For this review, take the finished solid that the model builds, in its own axes (mm). A direction names the side the tool comes from. Give positions to 0.01 mm unless a question says otherwise; leave off trailing zeros. Order: outer loops, then holes, each group sorted by start corner. A loop starts at its lowest first (then second) coordinate and runs counter-clockwise, first axis right, second up. Notation, with made-up numbers: (27.5, -2.5) - (73.5, -2.5) arc R31 ccw to (73.5, 22.5) - close; hole circle Ø7 at (57, 1.25). An arc over 180 degrees is marked (long way). Use a Markdown table: item, result. Add a question column.
1) We need section A-A on x = 0. Give the number of separate pieces and of enclosed holes in the cut face, then the cut area to 3 significant figures.
2) Clearance check with flat-ended pins moving along their axes: P1, Ø1.5, axis at x = 28, z = -6.5, coming from the -Y side; P2, Ø8, axis at y = -7.5, z = 19, coming from the +X side; P3, Ø2, axis at y = -4.5, z = 49.5, coming from the -X side. State where each tip first meets the part, or that it passes through.
3) Wall thickness on L1, parallel to Z at x = 0, y = -3; L2, parallel to X at y = -1.75, z = -24.5 (3 decimals); L3, parallel to Y at x = -19, z = -24.5: over which ranges is each line inside the solid? List them lowest first.
4) We need section B-B on z = 27.5. Write out the cut boundary in (x, y) (3 decimals).
5) Machinability: for faces 4 (the face through (41.275, -2, -1)), 5 (the face through (-23, -13, -12.7)), 6 (the face through (0, -3, -33.338)), which of the approach directions +Z, -Z, +X, -X, +Y, -Y give a long, thin tool a straight path to every point of the face, cutting with its end or side? Answer none if there is none.
6) We need section C-C on y = -9.5. Write out the cut boundary in (x, z), then the cut area to 3 significant figures.
7) Mouldability with a two-part tool opening along X and no side actions: class faces 1 (the face through (23.057, -23.872, 11.251)), 2 (the face through (19.837, -16, 0)), 3 (the face through (32.537, -21, 0)) as released by +X, released by -X, zero draft, split by the parting line, or undercut.
```python
from build123d import *

# Parameters (mm, degrees)
F0_W      = 82.55
F0_H      = 127
F0_R      = 2.3749
F0_W_2    = 6.35
F0_H_2    = 25.4
F0_W_3    = 33.3248
F0_H_3    = 66.675
F1_DEPTH  = 6.35
F2_R      = 3.175
F3_SIZE   = 1.5748
F4_SIZE   = 1.5748
F5_DEPTH  = 25.4
F6_DEPTH  = 25.4
F7_R      = 5.08
F8_R      = 5.08
F9_R      = 5.08
F10_R     = 1.5875
F11_DEPTH = 6.35
F12_R     = 1.5875
F13_DEPTH = 6.35


with BuildPart() as f1:
    # F0 (on Front) → F1 (new body)
    with BuildSketch(Plane.XZ):
        Rectangle(F0_W, F0_H)
        with Locations((0, -47.6123)):
            Circle(F0_R, mode=Mode.SUBTRACT)
        with Locations((-23.0124, 0)):
            Rectangle(F0_W_2, F0_H_2, mode=Mode.SUBTRACT)
        Rectangle(F0_W_3, F0_H_3, mode=Mode.SUBTRACT)
        with Locations((23.0124, 0)):
            Rectangle(F0_W_2, F0_H_2, mode=Mode.SUBTRACT)
        with Locations((0, 47.6123)):
            Circle(F0_R, mode=Mode.SUBTRACT)
    extrude(amount=F1_DEPTH)

    # F2
    f2_edges = [f1.edges().sort_by_distance(p)[0] for p in [
        (0, -6.35, 63.5),
        (41.275, -6.35, 0),
        (0, -6.35, -63.5),
        (-41.275, -6.35, 0),
    ]]
    fillet(f2_edges, radius=F2_R)

    # F3
    f3_edges = [f1.edges().sort_by_distance(p)[0] for p in [
        (-2.3749, -6.35, 47.6123),
    ]]
    chamfer(f3_edges, length=F3_SIZE)

    # F4
    f4_edges = [f1.edges().sort_by_distance(p)[0] for p in [
        (-2.3749, -6.35, -47.6123),
    ]]
    chamfer(f4_edges, length=F4_SIZE)

    # F0 (on Front) → F5 (join)
    with BuildSketch(Plane.XZ):
        with Locations((-23.0124, 0)):
            Rectangle(F0_W_2, F0_H_2)
    extrude(amount=F5_DEPTH)

    # F0 (on Front) → F6 (join)
    with BuildSketch(Plane.XZ):
        with Locations((23.0124, 0)):
            Rectangle(F0_W_2, F0_H_2)
    extrude(amount=F6_DEPTH)

    # F7
    f7_edges = [f1.edges().sort_by_distance(p)[0] for p in [
        (-23.0124, -25.4, 12.7),
    ]]
    fillet(f7_edges, radius=F7_R)

    # F8
    f8_edges = [f1.edges().sort_by_distance(p)[0] for p in [
        (23.0124, -25.4, 12.7),
        (-23.0124, -25.4, -12.7),
    ]]
    fillet(f8_edges, radius=F8_R)

    # F9
    f9_edges = [f1.edges().sort_by_distance(p)[0] for p in [
        (23.0124, -25.4, -12.7),
    ]]
    fillet(f9_edges, radius=F9_R)

    # F10 (on face) → F11 (join)
    with BuildSketch(Plane(origin=(-26.1874, 0, 0), x_dir=(0, -1, 0), z_dir=(-1, 0, 0))):
        with Locations((20.6375, 0)):
            Circle(F10_R)
    extrude(amount=F11_DEPTH)

    # F12 (on face) → F13 (join)
    with BuildSketch(Plane.YZ.offset(26.1874)):
        with Locations((-20.6375, 0)):
            Circle(F12_R)
    extrude(amount=F13_DEPTH)


solid = f1.part
```
Checked values:
| question | item | result |
|---|---|---|
| 1 | separate pieces | 4 |
| 1 | enclosed holes | 0 |
| 1 | area | 313 mm² |
| 2 | P1 | y = -6.35 |
| 2 | P2 | x = 41.26 |
| 2 | P3 | x = -41.26 |
| 3 | L1 | -63.5 to -49.99, -45.24 to -33.34, 33.34 to 45.24, 49.99 to 63.5 |
| 3 | L2 | -41.275 to -16.662, 16.662 to 41.275 |
| 3 | L3 | -6.35 to 0 |
| 4 | outline | (-41.275, -3.175) arc R3.175 ccw to (-38.1, -6.35) - (-16.662, -6.35) - (-16.662, 0) - (-41.275, 0) - close; (16.662, -6.35) - (38.1, -6.35) arc R3.175 ccw to (41.275, -3.175) - (41.275, 0) - (16.662, 0) - close |
| 5 | face 4 | +Z, -Z, +X, +Y, -Y |
| 5 | face 5 | -Z, +X, -X, -Y |
| 5 | face 6 | +Y, -Y |
| 6 | outline | (-26.19, -12.7) - (-19.84, -12.7) - (-19.84, 12.7) - (-26.19, 12.7) - close; (19.84, -12.7) - (26.19, -12.7) - (26.19, 12.7) - (19.84, 12.7) - close |
| 6 | area | 323 mm² |
| 7 | face 1 | zero draft |
| 7 | face 2 | undercut |
| 7 | face 3 | released by +X |
